Geometry check sheet. Reference: the model listing, model coordinates, mm. Face numbers are marked on the shaded views. Coordinates: 2 decimals unless noted, no trailing zeros. Write each loop counter-clockwise with the first axis right and the second up, starting at its lowest first coordinate (ties: lowest second). Pieces come first, ordered by that corner, then holes. Notation, with made-up numbers: M -23.75,-38 L 28.25,-38 A14 cw 28.25,-23 Z; hole C 20,72.5 d11. An arc over 180 degrees is marked long. Write each question's results on one line, items separated by ' | '.
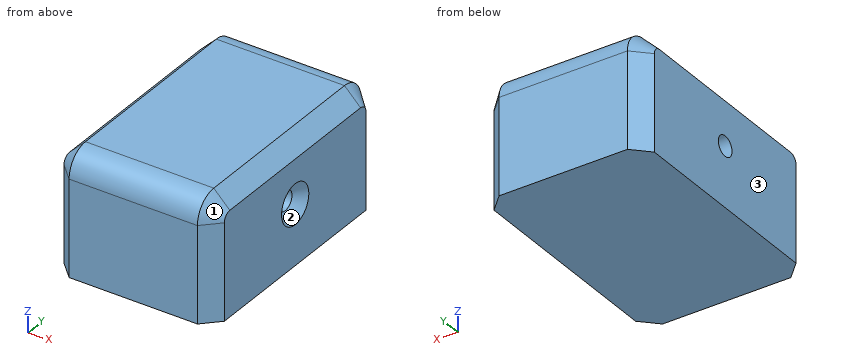
```python
from build123d import *

# Parameters (mm, degrees)
F0_W           = 50.8
F0_H           = 38.1
F1_DEPTH       = 76.2
F2_R           = 7.62
F3_SIZE        = 5.08
F5_D           = 6.35
F5_CSINK_D     = 12.7
F5_CSINK_ANGLE = 90


with BuildPart() as f1:
    # F0 (on Front) → F1 (new body)
    with BuildSketch(Plane.XZ):
        with Locations((25.4, 19.05)):
            Rectangle(F0_W, F0_H)
    extrude(amount=F1_DEPTH)

    # F2
    f2_edges = [f1.edges().sort_by_distance(p)[0] for p in [
        (25.4, -76.2, 38.1),
        (25.4, 0, 38.1),
    ]]
    fillet(f2_edges, radius=F2_R)

    # F3
    f3_edges = [f1.edges().sort_by_distance(p)[0] for p in [
        (50.8, -38.1, 38.1),
        (0, -38.1, 38.1),
    ]]
    chamfer(f3_edges, length=F3_SIZE)

    # F5 (through all)
    with Locations(Plane.YZ.offset(50.8)):
        with Locations((-38.1, 19.05)):
            CounterSinkHole(F5_D / 2, F5_CSINK_D / 2, counter_sink_angle=F5_CSINK_ANGLE)


solid = f1.part
```
Q1. Mould release check, pull along Y, two halves, no side actions. Record for the marked faces 1, 2 and 3: pulls with the +Y half, pulls with the -Y half, needs draft (parallel to the pull), parting line crosses it, or undercut.
Geometry check:
face 1: pulls with the -Y half | face 2: undercut | face 3: needs draft
Q2. Sectioned sample at A-A on z = 19.05. Record the cut outline in (x, y) (3 decimals), and give its area (3 significant figures).
Geometry check:
outline: M 0,-71.12 L 5.08,-76.2 L 45.72,-76.2 L 50.8,-71.12 L 50.8,-44.45 L 47.625,-41.275 L 0,-41.275 Z; M 0,-34.925 L 47.625,-34.925 L 50.8,-31.75 L 50.8,-5.08 L 45.72,0 L 5.08,0 L 0,-5.08 Z | area: 3,490 mm2
Q3. Sectioned sample at C-C on x = 24. Record the cut outline in (y, z) (3 decimals), and give its area (3 significant figures).
Geometry check:
outline: M -76.2,0 L 0,0 L 0,30.48 A7.62 ccw -7.62,38.1 L -68.58,38.1 A7.62 ccw -76.2,30.48 Z; hole C -38.1,19.05 d6.35 | area: 2,850 mm2
Q4. Sectioned sample at B-B on y = -38.1. Record the cut outline in (x, z) (3 decimals).
Geometry check:
outline: M 0,0 L 50.8,0 L 50.8,12.7 L 47.625,15.875 L 0,15.875 Z; M 0,22.225 L 47.625,22.225 L 50.8,25.4 L 50.8,33.02 L 45.72,38.1 L 5.08,38.1 L 0,33.02 Z
Q5. Scan lines: probe 1 along Z at (x, y) = (23, -38); probe 2 along Y at (x, z) = (30, 18.5); probe 3 along Y at (x, z) = (46.5, 21.5). Record each from-to range of solid material in increasing order.
Geometry check:
probe 1: z = 0 to 15.88, 22.22 to 38.1 | probe 2: y = -76.2 to -41.23, -34.97 to 0 | probe 3: y = -75.42 to -40.12, -36.08 to -0.78
